For this review, take the finished solid that the model builds, in its own axes (mm). Face numbers are marked on the shaded views. Coordinates: 2 decimals unless noted, no trailing zeros. Write each loop counter-clockwise with the first axis right and the second up, starting at its lowest first coordinate (ties: lowest second). Pieces come first, ordered by that corner, then holes. Notation, with made-up numbers: M -37,66 L -15,66 A24 ccw -15,81 Z; hole C -19.5,-11.75 d6. An arc over 180 degrees is marked long. Return JSON: item names as keys, results as strings.
```python
from build123d import *

# Parameters (mm, degrees)
SKETCH_1_W          = 10
SKETCH_1_H          = 10
SKETCH_1_W_2        = 8
SKETCH_1_H_2        = 8
EXTRUDE_1_DEPTH     = 60
CUT_EXTRUDE_1_REACH = 63.644
SKETCH_2_R          = 2.1
CUT_EXTRUDE_2_REACH = 63.644
SKETCH_3_R          = 2.15


with BuildPart() as part:
    # ｽｹｯﾁ1 → 押し出し-薄板1 (new body)
    with BuildSketch(Plane.XY):
        with Locations((5, 5)):
            Rectangle(SKETCH_1_W, SKETCH_1_H)
        with Locations((5, 5)):
            Rectangle(SKETCH_1_W_2, SKETCH_1_H_2, mode=Mode.SUBTRACT)
    extrude(amount=EXTRUDE_1_DEPTH)

    # ｶｯﾄ - 押し出し1: up to this face of the body (flat: up to its plane)
    cut_extrude_1_end = Plane(part.part.faces().sort_by_distance((0, 5, 30))[0])
    # ｽｹｯﾁ2 → ｶｯﾄ - 押し出し1 (cut, up to the picked face)
    with BuildSketch(Plane(origin=(10, 0, 0), x_dir=(0, 0, -1), z_dir=(1, 0, 0)), mode=Mode.PRIVATE) as cut_extrude_1_sk1:
        with Locations(Location((-55, 5, 0), (0, 0, 90))):
            Circle(SKETCH_2_R)
    cut_extrude_1_tool1 = split(extrude(cut_extrude_1_sk1.sketch, amount=-CUT_EXTRUDE_1_REACH, mode=Mode.PRIVATE), bisect_by=cut_extrude_1_end, keep=Keep.BOTH, mode=Mode.PRIVATE)
    # ｽｹｯﾁ2 → ｶｯﾄ - 押し出し1 (cut, up to the picked face)
    with BuildSketch(Plane(origin=(10, 0, 0), x_dir=(0, 0, -1), z_dir=(1, 0, 0)), mode=Mode.PRIVATE) as cut_extrude_1_sk2:
        with Locations(Location((-5, 5, 0), (0, 0, 270))):
            Circle(SKETCH_2_R)
    cut_extrude_1_tool2 = split(extrude(cut_extrude_1_sk2.sketch, amount=-CUT_EXTRUDE_1_REACH, mode=Mode.PRIVATE), bisect_by=cut_extrude_1_end, keep=Keep.BOTH, mode=Mode.PRIVATE)
    add(cut_extrude_1_tool1.solids().sort_by(Axis((10, 5, 55), (-1, 0, 0)))[0], mode=Mode.SUBTRACT)
    add(cut_extrude_1_tool2.solids().sort_by(Axis((10, 5, 5), (-1, 0, 0)))[0], mode=Mode.SUBTRACT)

    # ｶｯﾄ - 押し出し2: up to this face of the body (flat: up to its plane)
    cut_extrude_2_end = Plane(part.part.faces().sort_by_distance((5, 0, 30))[0])
    # ｽｹｯﾁ3 → ｶｯﾄ - 押し出し2 (cut, up to the picked face)
    with BuildSketch(Plane(origin=(0, 10, 0), x_dir=(1, 0, 0), z_dir=(0, 1, 0)), mode=Mode.PRIVATE) as cut_extrude_2_sk1:
        with Locations(Location((5, -30, 0), (0, 0, 270))):
            Circle(SKETCH_3_R)
    cut_extrude_2_tool1 = split(extrude(cut_extrude_2_sk1.sketch, amount=-CUT_EXTRUDE_2_REACH, mode=Mode.PRIVATE), bisect_by=cut_extrude_2_end, keep=Keep.BOTH, mode=Mode.PRIVATE)
    add(cut_extrude_2_tool1.solids().sort_by(Axis((5, 10, 30), (0, -1, 0)))[0], mode=Mode.SUBTRACT)


solid = part.part
```
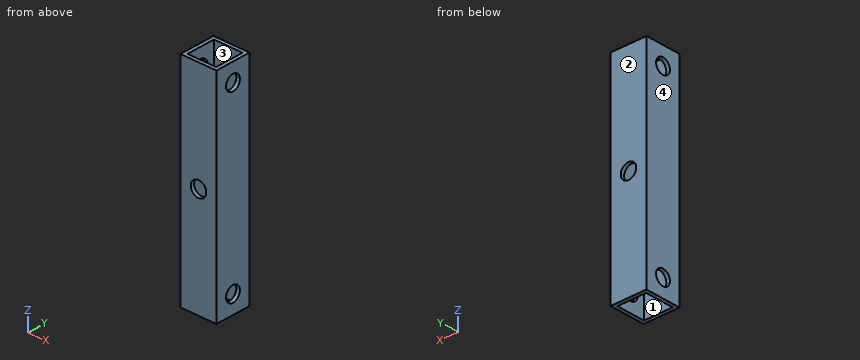
1. We need section A-A (x = 5). State the section outline as (y, z) points.
Checks:
{"outline": "M 0,0 L 1,0 L 1,27.85 L 0,27.85 Z; M 0,32.15 L 1,32.15 L 1,60 L 0,60 Z; M 9,0 L 10,0 L 10,27.85 L 9,27.85 Z; M 9,32.15 L 10,32.15 L 10,60 L 9,60 Z"}
2. Wall thickness on L1, parallel to Z at x = 0.45, y = 5; L2, parallel to X at y = 7, z = 10.5: over which ranges is each line inside the solid? List them lowest first. Write a range as from..to.
Checks:
{"L1": "0..2.9, 7.1..52.9, 57.1..60", "L2": "0..1, 9..10"}
3. We need section C-C (y = 2). State the section outline as (x, z) points.
Checks:
{"outline": "M 0,0 L 1,0 L 1,60 L 0,60 Z; M 9,0 L 10,0 L 10,60 L 9,60 Z"}
4. Draft analysis for pull direction Y (two halves, no side actions). For the marked faces 1, 2, 3 and 4, state which applies: +Y half, -Y half, draft (parallel to the pull), parting line (faces both ways), or undercut.
Checks:
{"face 1": "undercut", "face 2": "+Y half", "face 3": "undercut", "face 4": "draft"}
5. We need section D-D (z = 44.5). State the section outline as (x, y) points, plus the area to 3 significant figures.
Checks:
{"outline": "M 0,0 L 10,0 L 10,10 L 0,10 Z; hole M 1,1 L 9,1 L 9,9 L 1,9 Z", "area": "36.0 mm2"}
6. We need section B-B (z = 30). State the section outline as (x, y) points, plus the area to 3 significant figures.
Checks:
{"outline": "M 0,0 L 2.85,0 L 2.85,1 L 1,1 L 1,9 L 2.85,9 L 2.85,10 L 0,10 Z; M 7.15,0 L 10,0 L 10,10 L 7.15,10 L 7.15,9 L 9,9 L 9,1 L 7.15,1 Z", "area": "27.4 mm2"}
